```python
from build123d import *

# Parameters (mm, degrees)
BOSS_EXTRU_1_DEPTH      = 682
ENL_V_MAT_EXTRU_1_DEPTH = 590
ENL_V_MAT_EXTRU_2_DEPTH = 590


with BuildPart() as part:
    # Esquisse1 → Boss.-Extru.1 (new body)
    with BuildSketch(Plane(origin=(0, 0, 0), x_dir=(1, 0, 0), z_dir=(0, 1, 0))):
        Polygon((-20, 20.113636364), (20, 20.113636364), (20, 18.113636364), (-18, 18.113636364), (-18, -19.886363636), (-20, -19.886363636), align=None)
    extrude(amount=BOSS_EXTRU_1_DEPTH)

    # Esquisse2 → Enlèv. mat.-Extru.1 (cut)
    with BuildSketch(Plane(origin=(0, 0, -20.113636364), x_dir=(-1, 0, 0), z_dir=(0, 0, -1))):
        Polygon((20, 0), (-20, 40), (-20, 0), align=None)
    extrude(amount=-ENL_V_MAT_EXTRU_1_DEPTH, mode=Mode.SUBTRACT)

    # Esquisse3 → Enlèv. mat.-Extru.2 (cut)
    with BuildSketch(Plane.ZY.offset(20)):
        Polygon((-20.113636364, 0), (19.886363636, 40), (19.886363636, 0), align=None)
    extrude(amount=-ENL_V_MAT_EXTRU_2_DEPTH, mode=Mode.SUBTRACT)


solid = part.part
```
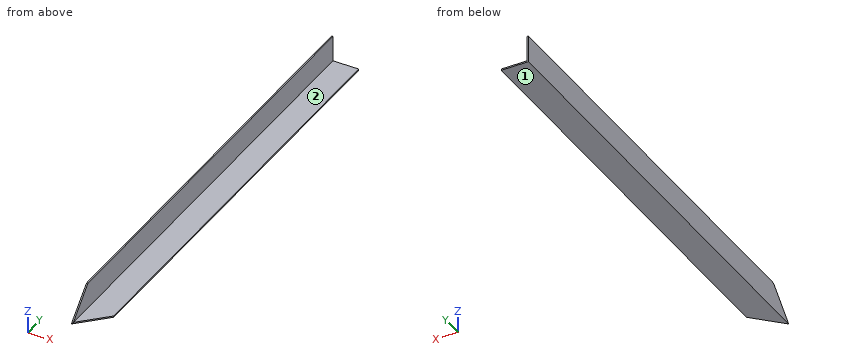
Here's how the part is built. I have some questions about the finished solid (model axes, mm). Face numbers are marked on the shaded views. A direction names the side the tool comes from. Coordinates: 2 decimals unless noted, no trailing zeros. Write each loop counter-clockwise with the first axis right and the second up, starting at its lowest first coordinate (ties: lowest second). Pieces come first, ordered by that corner, then holes. Notation, with made-up numbers: (47, 73.25) -> (71, 73.25) arc R26 ccw to (71, 97.25) -> close; hole circle Ø5 at (-17, 60). An arc over 180 degrees is marked (long way). Use a Markdown table: item, result. Add a question column.
(1) I'm going to push flat-ended pins straight in: P1, Ø2, axis at x = 5, y = 208, coming from the +Z side; P2, Ø4, axis at y = 566, z = -15, coming from the +X side. Where does each tip first touch, or does it pass through?
(2) For the marked faces 1 and 2, which set-ups out of +Z, -Z, +X, -X, +Y, -Y let a thin tool reach every point of the face, with its end or its side?
(3) If we section it at B-B, the plane x = -3.5: Write out the boundary of the cut face in (y, z), and give its area (3 significant figures).
(4) If we section it at C-C, the plane z = 11: Write out the boundary of the cut face in (x, y), and give its area (3 significant figures).
(5) Please list where these lines run through material, in increasing order: line 1 (X direction, y = 282, z = -1); line 2 (Z direction, x = -14, y = 530).
(6) If we section it at A-A, the plane y = 614.5: Write out the boundary of the cut face in (x, z).
Outcome:
| question | item | result |
|---|---|---|
| 1 | P1 | stops at z = -18.11 |
| 1 | P2 | stops at x = -18 |
| 2 | face 1 | -Z, +X, -X, +Y, -Y |
| 2 | face 2 | +Z, +X, +Y, -Y |
| 3 | outline | (16.5, -20.11) -> (682, -20.11) -> (682, -18.11) -> (16.5, -18.11) -> close |
| 3 | area | 1,330 mm^2 |
| 4 | outline | (-20, 31.11) -> (-18, 31.11) -> (-18, 682) -> (-20, 682) -> close |
| 4 | area | 1,300 mm^2 |
| 5 | line 1 | x = -20 to -18 |
| 5 | line 2 | z = -20.11 to -18.11 |
| 6 | outline | (-20, -20.11) -> (20, -20.11) -> (20, -18.11) -> (-18, -18.11) -> (-18, 19.89) -> (-20, 19.89) -> close |
